Input: dimensioned drawing with shaded views. Units: mm. Origin: part minimum x, y, z. A direction names the side the tool comes from. Round coordinates to 2 decimals unless told otherwise and drop trailing zeros. Loops run counter-clockwise (first coordinate to the right, second up) from the corner with the lowest first, then second, coordinate; pieces in that order, holes last. Notation, with made-up numbers: (54, -3.5) - (66, -3.5) arc R6 ccw to (66, 3.5) - close; hole circle Ø4 at (31.5, 69.5). An arc over 180 degrees is marked (long way). Write each question's results on one line, items separated by ' | '.
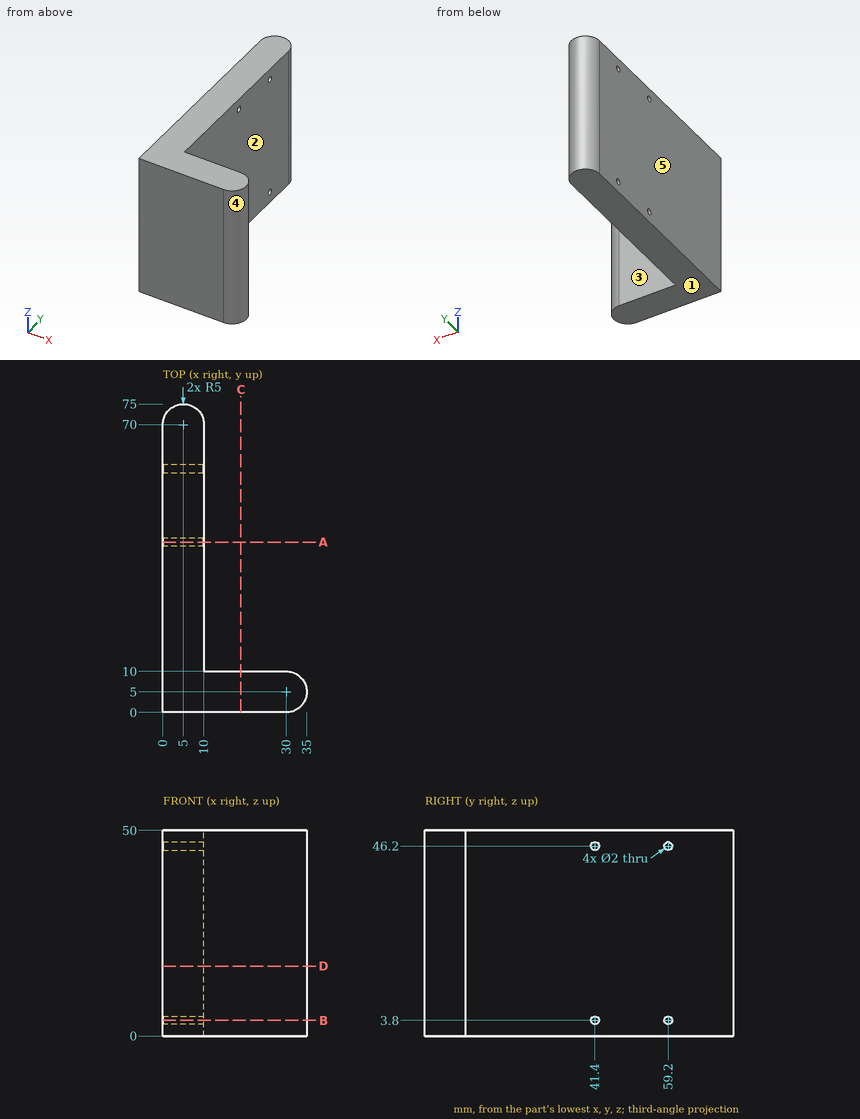
1. Section query B-B, the plane z = 3.8. Output: boundary loops of the cut face in (x, y), plus the area to 3 significant figures.
Answer:
outline: (0, 0) - (30, 0) arc R5 ccw to (30, 10) - (10, 10) - (10, 40.4) - (0, 40.4) - close; (0, 42.4) - (10, 42.4) - (10, 58.2) - (0, 58.2) - close; (0, 60.2) - (10, 60.2) - (10, 70) arc R5 ccw to (0, 70) - close | area: 939 mm^2
2. Section query C-C, the plane x = 19. Output: boundary loops of the cut face in (y, z).
Answer:
outline: (0, 0) - (10, 0) - (10, 50) - (0, 50) - close
3. Section query A-A, the plane y = 41.4. Output: boundary loops of the cut face in (x, z).
Answer:
outline: (0, 0) - (10, 0) - (10, 2.8) - (0, 2.8) - close; (0, 4.8) - (10, 4.8) - (10, 45.2) - (0, 45.2) - close; (0, 47.2) - (10, 47.2) - (10, 50) - (0, 50) - close
4. Contact query for a flat-ended pin moving along its axis: pin 1 (12 mm diameter, centred on y = 41, z = 38.5, fed in from +X). Output: stop coordinate, or through.
Answer:
pin 1: x = 10
5. Section query D-D, the plane z = 17. Output: boundary loops of the cut face in (x, y).
Answer:
outline: (0, 0) - (30, 0) arc R5 ccw to (30, 10) - (10, 10) - (10, 70) arc R5 ccw to (0, 70) - close
6. Mould query, pull axis X, two halves, no side actions, for the marked faces 3, 4 and 5. Classes: pulls with the +X half, pulls with the -X half, needs draft (parallel to the pull), parting line crosses it, or undercut.
Answer:
face 3: needs draft | face 4: pulls with the +X half | face 5: pulls with the -X half
7. Set-up query: the marked faces 1 and 2. Return all of +Z, -Z, +X, -X, +Y, -Y with unobstructed straight access to the full face (end or side cutting, diameter ignored); none if empty.
Answer:
face 1: -Z, +X, -X, +Y, -Y | face 2: +Z, -Z, +X, +Y
8. Line query: line 1 (Z direction, x = 3.5, y = 59.2); line 2 (Y direction, x = 3, z = 3.8); line 3 (Z direction, x = 3, y = 41). Output: solid intervals per line, ascending. Write a range as [from, to].
Answer:
line 1: [0, 2.8], [4.8, 45.2], [47.2, 50] | line 2: [0, 40.4], [42.4, 58.2], [60.2, 74.58] | line 3: [0, 2.88], [4.72, 45.28], [47.12, 50]
